Design review of the part built by this model. Coordinates are the model's own, in mm. Face numbers are marked on the shaded views. A direction names the side the tool comes from. Give positions to 0.01 mm unless a question says otherwise; leave off trailing zeros. Loops run counter-clockwise (first coordinate to the right, second up) from the corner with the lowest first, then second, coordinate; pieces in that order, holes last. Notation, with made-up numbers: (15.5, -15.5) - (37.5, -15.5) arc R21 ccw to (37.5, 14.5) - close; hole circle Ø11 at (-17.5, 66.5). An arc over 180 degrees is marked (long way). Write each question's results on one line, items separated by ' | '.
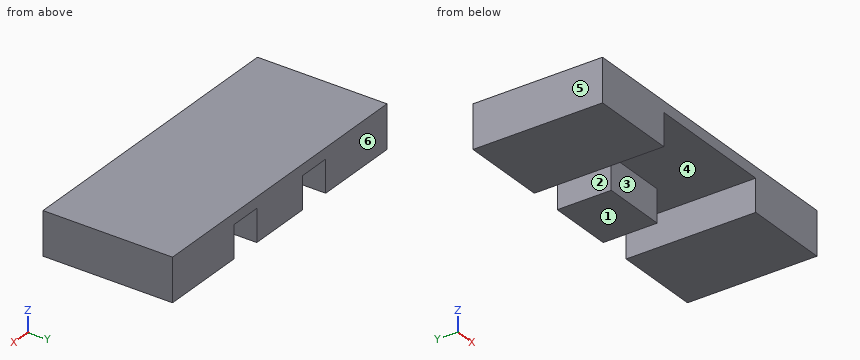
```python
from build123d import *

# Parameters (mm, degrees)
SKETCH_1_W      = 280
SKETCH_1_H      = 120
EXTRUDE_1_DEPTH = 10
SKETCH_2_W      = 60
SKETCH_2_H      = 50
EXTRUDE_2_DEPTH = 30
SKETCH_3_W      = 80
SKETCH_3_H      = 120
EXTRUDE_3_DEPTH = 30


with BuildPart() as part:
    # 스케치1 → 보스-돌출1 (new body)
    with BuildSketch(Plane.XY):
        Rectangle(SKETCH_1_W, SKETCH_1_H)
    extrude(amount=EXTRUDE_1_DEPTH)

    # 스케치2 → 보스-돌출2 (add)
    with BuildSketch(Plane(origin=(0, 0, 0), x_dir=(-1, 0, 0), z_dir=(0, 0, -1))):
        with Locations((0, 35)):
            Rectangle(SKETCH_2_W, SKETCH_2_H)
    extrude(amount=EXTRUDE_2_DEPTH)

    # 스케치3 → 보스-돌출3 (add)
    with BuildSketch(Plane(origin=(0, 0, 0), x_dir=(-1, 0, 0), z_dir=(0, 0, -1))):
        with Locations((-100, 0)):
            Rectangle(SKETCH_3_W, SKETCH_3_H)
        with Locations((100, 0)):
            Rectangle(SKETCH_3_W, SKETCH_3_H)
    extrude(amount=EXTRUDE_3_DEPTH)


solid = part.part
```
Item 1: Clearance check with a flat-ended pin moving along its axis: P1, Ø9, axis at x = 12.5, z = -17, coming from the -Y side. State where the tip first meets the part, or that it passes through.
Output values:
P1: stops at y = 10
Item 2: Tool access review of the marked faces 1 and 2: name each direction out of +Z, -Z, +X, -X, +Y, -Y from which nothing blocks a thin tool from reaching the whole face with its end or side.
Output values:
face 1: -Z, +X, -X, +Y, -Y | face 2: -Z, +Y, -Y
Item 3: Wall thickness on probe 1 along X at (y, z) = (23, -28); probe 2 along X at (y, z) = (-31, -21); probe 3 along Z at (x, y) = (-52.5, -8.5): over which ranges is each line inside the solid? List them lowest first.
Output values:
probe 1: x = -140 to -60, -30 to 30, 60 to 140 | probe 2: x = -140 to -60, 60 to 140 | probe 3: z = 0 to 10
Item 4: We need section D-D on y = -17. Give the boundary of the cut face in (x, z).
Output values:
outline: (-140, -30) - (-60, -30) - (-60, 0) - (60, 0) - (60, -30) - (140, -30) - (140, 10) - (-140, 10) - close
Item 5: We need section C-C on x = -6. Give the boundary of the cut face in (y, z), then the cut area to 3 significant figures.
Output values:
outline: (-60, 0) - (10, 0) - (10, -30) - (60, -30) - (60, 10) - (-60, 10) - close | area: 2,700 mm²
Item 6: We need section B-B on y = 41. Give the boundary of the cut face in (x, z), then the cut area to 3 significant figures.
Output values:
outline: (-140, -30) - (-60, -30) - (-60, 0) - (-30, 0) - (-30, -30) - (30, -30) - (30, 0) - (60, 0) - (60, -30) - (140, -30) - (140, 10) - (-140, 10) - close | area: 9,400 mm²
Item 7: Draft analysis for pull direction X (two halves, no side actions). For the marked faces 3, 4, 5 and 6, state which applies: +X half, -X half, draft (parallel to the pull), parting line (faces both ways), or undercut.
Output values:
face 3: undercut | face 4: undercut | face 5: -X half | face 6: draft
Item 8: We need section A-A on z = -5.5. Give the boundary of the cut face in (x, y).
Output values:
outline: (-140, -60) - (-60, -60) - (-60, 60) - (-140, 60) - close; (-30, 10) - (30, 10) - (30, 60) - (-30, 60) - close; (60, -60) - (140, -60) - (140, 60) - (60, 60) - close
